```python
from build123d import *

# Parameters (mm, degrees)
SKETCH1_R                = 75
BOSS_EXTRUDE1_DEPTH      = 15
BOSS_EXTRUDE2_DEPTH      = 80
CUT_EXTRUDE1_START       = -15
CUT_EXTRUDE1_DEPTH       = 15
F_4_0_MM_DOWEL_HOLES1_D  = 4
FILLET1_R                = 4
FILLET2_R                = 4
CIRPATTERN1_COUNT        = 3
FILLET1_OF_CIRPATTERN1_R = 4
FILLET2_OF_CIRPATTERN1_R = 4


with BuildPart() as part:
    # Sketch1 → Boss-Extrude1 (new body)
    with BuildSketch(Plane(origin=(0, 0, 0), x_dir=(1, 0, 0), z_dir=(0, 1, 0))):
        with Locations(Location((0, 0, 0), (0, 0, 270))):
            Circle(SKETCH1_R)
    extrude(amount=BOSS_EXTRUDE1_DEPTH)

    # Sketch2 → Boss-Extrude2 (add)
    with BuildSketch(Plane(origin=(0, 15, 0), x_dir=(1, 0, 0), z_dir=(0, 1, 0))):
        with BuildLine():
            Line((-25, 70.710678119), (-25, 62.710678119))
            Line((-25, 62.710678119), (25, 62.710678119))
            Line((25, 62.710678119), (25, 70.710678119))
            ThreePointArc((25, 70.710678119), (0, 75), (-25, 70.710678119))
        make_face()
    boss_extrude2 = extrude(amount=BOSS_EXTRUDE2_DEPTH)

    # Sketch3 → Cut-Extrude1 (cut)
    with BuildSketch(Plane(origin=(0, 95, 0), x_dir=(1, 0, 0), z_dir=(0, 1, 0)).offset(CUT_EXTRUDE1_START)):
        with BuildLine():
            Line((-20, 72.284161474), (-20, 62.710678119))
            Line((-20, 62.710678119), (20, 62.710678119))
            Line((20, 62.710678119), (20, 72.284161474))
            ThreePointArc((20, 72.284161474), (0, 75), (-20, 72.284161474))
        make_face()
    cut_extrude1 = extrude(amount=CUT_EXTRUDE1_DEPTH, mode=Mode.SUBTRACT)

    # Ø4.0 mm Dowel Holes1 (through all)
    with Locations(Plane(origin=(25, 0, 0), x_dir=(0, 0, -1), z_dir=(1, 0, 0))):
        with Locations((66.710678119, 91)):
            f_4_0_mm_dowel_holes1 = Hole(F_4_0_MM_DOWEL_HOLES1_D / 2)

    # Fillet1
    fillet1_edges = [part.edges().sort_by_distance(p)[0] for p in [
        (22.5, 95, -62.710678119),
        (-22.5, 95, -62.710678119),
    ]]
    fillet(fillet1_edges, radius=FILLET1_R)

    # Fillet2
    fillet2_edges = [part.edges().sort_by_distance(p)[0] for p in [
        (20, 80, -67.497419796),
        (-20, 80, -67.497419796),
    ]]
    fillet(fillet2_edges, radius=FILLET2_R)

    # CirPattern1: Boss-Extrude2, Cut-Extrude1, Ø4.0 mm Dowel Holes1 ×3 about axis
    cirpattern1_axis = Axis((0, 0, 0), (0, 1, 0))
    add([boss_extrude2.rotate(cirpattern1_axis, i * 360 / CIRPATTERN1_COUNT) for i in range(1, CIRPATTERN1_COUNT)])
    add([cut_extrude1.rotate(cirpattern1_axis, i * 360 / CIRPATTERN1_COUNT) for i in range(1, CIRPATTERN1_COUNT)], mode=Mode.SUBTRACT)
    add([f_4_0_mm_dowel_holes1.rotate(cirpattern1_axis, i * 360 / CIRPATTERN1_COUNT) for i in range(1, CIRPATTERN1_COUNT)], mode=Mode.SUBTRACT)

    # Fillet1 of CirPattern1
    fillet1_of_cirpattern1_edges = [part.edges().sort_by_distance(p)[0] for p in [
        (-65.559040339, 95, 11.869767474),
        (-43.059040339, 95, 50.840910644),
        (43.059040339, 95, 50.840910644),
        (65.559040339, 95, 11.869767474),
    ]]
    fillet(fillet1_of_cirpattern1_edges, radius=FILLET1_OF_CIRPATTERN1_R)

    # Fillet2 of CirPattern1
    fillet2_of_cirpattern1_edges = [part.edges().sort_by_distance(p)[0] for p in [
        (-68.454480234, 80, 16.428201822),
        (-48.454480234, 80, 51.069217974),
        (48.454480234, 80, 51.069217974),
        (68.454480234, 80, 16.428201822),
    ]]
    fillet(fillet2_of_cirpattern1_edges, radius=FILLET2_OF_CIRPATTERN1_R)


solid = part.part
```
Input: part model. Units: mm. Frame: model coordinates. A direction names the side the tool comes from. Round coordinates to 2 decimals unless told otherwise and drop trailing zeros. Order: outer loops, then holes, each group sorted by start corner. A loop starts at its lowest first (then second) coordinate and runs counter-clockwise, first axis right, second up. Notation, with made-up numbers: (-29.5, 61.25) - (-6.5, 61.25) arc R16 cw to (-6.5, 91.25) - close; hole circle Ø8 at (59, 86.5). An arc over 180 degrees is marked (long way). One line per question, with ' | ' between items. Start each with the question number.
1) Cut plane C-C, the plane x = 0. Return the cut outline in (y, z).
2) Cut plane B-B, the plane z = 0. Return the cut outline in (x, y), then the cut area to 3 significant figures.
3) Contact query for flat-ended pins moving along their axis: P1, Ø10.5, axis at y = 88.5, z = -69.5, coming from the -X side; P2, Ø3, axis at y = 88, z = -68.5, coming from the +X side; P3, Ø10, axis at x = 56.5, y = 83.5, coming from the +Z side. Output: stop coordinate, or through.
4) Cut plane D-D, the plane y = 10. Return the cut outline in (x, z), then the cut area to 3 significant figures.
5) Ray query, probe 1 along Z at (x, y) = (-20, 26); probe 2 along Y at (x, z) = (-38.5, 58.5); probe 3 along X at (y, z) = (78, 12). Return the intervals inside material, ascending.
6) Cut plane A-A, the plane y = 21. Return the cut outline in (x, z), then the cut area to 3 significant figures.
7) Pull-direction query (Z, two-part tool) for faces 1 (the flat face through (70.32, 54.44, 11.73)), 2 (the flat face through (-48, 95, 54)), 3 (the cylindrical face through (-69, 93, 14)), 4 (the cylindrical face through (-46.731, 92.983, 53.001)); classes: +Z half, -Z half, draft (parallel to the pull), parting line (faces both ways), or undercut.
8) Set-up query: faces 5 (the flat face through (-68.396, 88.201, 16.395)), 6 (the cylindrical face through (-18.859, 81.203, -67.918)), 7 (the cylindrical face through (66.53, 93.8, 12.47)). Return all of +Z, -Z, +X, -X, +Y, -Y with unobstructed straight access to the full face (end or side cutting, diameter ignored); none if empty.
Worked out:
1) outline: (0, -75) - (80, -75) - (80, -62.71) - (15, -62.71) - (15, 75) - (0, 75) - close
2) outline: (-75, 0) - (75, 0) - (75, 15) - (-75, 15) - close | area: 2,250 mm^2
3) P1: stops at x = -25 | P2: stops at x = 25 | P3: stops at z = 54.52
4) outline: circle Ø150 at (0, 0) | area: 17,700 mm^2
5) probe 1: z = -72.28 to -62.71 | probe 2: y = 0 to 15 | probe 3: x = -70.78 to -65.48, 65.48 to 70.78
6) outline: (-73.74, 13.7) - (-66.81, 9.7) - (-41.81, 53.01) - (-48.74, 57.01) arc R75 ccw to start; (-25, -70.71) arc R75 ccw to (25, -70.71) - (25, -62.71) - (-25, -62.71) - close; (41.81, 53.01) - (66.81, 9.7) - (73.74, 13.7) arc R75 ccw to (48.74, 57.01) - close | area: 1,630 mm^2
7) face 1: -Z half | face 2: draft | face 3: undercut | face 4: undercut
8) face 5: +Z, +Y | face 6: +Z, -Z, +Y | face 7: -Z, +Y
